Can you work these out from the model? Positions are in its coordinate system, mm. A direction names the side the tool comes from. Give positions to 0.01 mm unless a question says otherwise; leave off trailing zeros. Order: outer loops, then holes, each group sorted by start corner. A loop starts at its lowest first (then second) coordinate and runs counter-clockwise, first axis right, second up. Notation, with made-up numbers: (-5.5, -15) - (46.5, -15) arc R10 ccw to (46.5, -11) - close; hole circle Ø2 at (43, -15). An arc over 180 degrees is marked (long way). Return JSON: item names as keys, results as strings.
```python
from build123d import *

# Parameters (mm, degrees)
SKETCH_W      = 50
SKETCH_H      = 53
PAD_DEPTH     = 3
SKETCH001_W   = 50
SKETCH001_H   = 3
PAD001_DEPTH  = 48
SKETCH002_R   = 11.05
SKETCH002_R_2 = 1.75
POCKET_DEPTH  = 53.001
FILLET_R      = 2
CHAMFER_SIZE  = 5


with BuildPart() as part:
    # Sketch → Pad (new body)
    with BuildSketch(Plane.XY):
        Rectangle(SKETCH_W, SKETCH_H)
        with BuildLine():
            ThreePointArc((-17.1, -15.5), (-15, -17.6), (-12.9, -15.5))
            Line((-12.9, -15.5), (-12.9, 14.5))
            ThreePointArc((-12.9, 14.5), (-15, 16.6), (-17.1, 14.5))
            Line((-17.1, -15.5), (-17.1, 14.5))
        make_face(mode=Mode.SUBTRACT)
        with BuildLine():
            ThreePointArc((12.9, -15.5), (15, -17.6), (17.1, -15.5))
            Line((17.1, -15.5), (17.1, 14.5))
            ThreePointArc((17.1, 14.5), (15, 16.6), (12.9, 14.5))
            Line((12.9, -15.5), (12.9, 14.5))
        make_face(mode=Mode.SUBTRACT)
    extrude(amount=PAD_DEPTH)

    # Sketch001 → Pad001 (new body)
    with BuildSketch(Plane.XY.offset(3)):
        with Locations((0, 25)):
            Rectangle(SKETCH001_W, SKETCH001_H)
    extrude(amount=PAD001_DEPTH)

    # Sketch002 → Pocket (cut, through all)
    with BuildSketch(Plane(origin=(0, 26.5, 0), x_dir=(-1, 0, 0), z_dir=(0, 1, 0))):
        with Locations((0, 30)):
            Circle(SKETCH002_R)
        with Locations((-15.5, 45.5)):
            Circle(SKETCH002_R_2)
        with Locations((15.5, 45.5)):
            Circle(SKETCH002_R_2)
        with Locations((-15.5, 14.5)):
            Circle(SKETCH002_R_2)
        with Locations((15.5, 14.5)):
            Circle(SKETCH002_R_2)
    extrude(amount=-POCKET_DEPTH, mode=Mode.SUBTRACT)

    # Fillet
    fillet_edges = [part.edges().sort_by_distance(p)[0] for p in [
        (0, 26.5, 0),
        (0, 23.5, 3),
    ]]
    fillet(fillet_edges, radius=FILLET_R)

    # Chamfer
    chamfer_edges = [part.edges().sort_by_distance(p)[0] for p in [
        (25, 25, 51),
        (-25, 25, 51),
        (-25, -26.5, 1.5),
        (25, -26.5, 1.5),
    ]]
    chamfer(chamfer_edges, length=CHAMFER_SIZE)


solid = part.part
```
1. Suppose I cut it at D-D (x = 12). List the corners of the cut face in (y, z) for me.
Checks:
{"outline": "(-26.5, 0) - (24.5, 0) arc R2 ccw to (26.5, 2) - (26.5, 51) - (23.5, 51) - (23.5, 5) arc R2 cw to (21.5, 3) - (-26.5, 3) - close"}
2. Thinking about a two-plate mould opening in Z: for faces 1 (the face through (23, 25, 48)), 2 (the face through (-15, 16.6, 1.5)), 3 (the face through (-15.12, 25.02, 43.79)), which applies, +Z half, -Z half, draft (parallel to the pull), parting line (faces both ways), or undercut?
Checks:
{"face 1": "+Z half", "face 2": "draft", "face 3": "undercut"}
3. Suppose I cut it at B-B (y = 2.5). List the corners of the cut face in (x, z) for me.
Checks:
{"outline": "(-25, 0) - (-17.1, 0) - (-17.1, 3) - (-25, 3) - close; (-12.9, 0) - (12.9, 0) - (12.9, 3) - (-12.9, 3) - close; (17.1, 0) - (25, 0) - (25, 3) - (17.1, 3) - close"}
4. Suppose I cut it at C-C (z = 14.5). List the corners of the cut face in (x, y) for me, plus the area to 3 significant figures.
Checks:
{"outline": "(-25, 23.5) - (-17.25, 23.5) - (-17.25, 26.5) - (-25, 26.5) - close; (-13.75, 23.5) - (13.75, 23.5) - (13.75, 26.5) - (-13.75, 26.5) - close; (17.25, 23.5) - (25, 23.5) - (25, 26.5) - (17.25, 26.5) - close", "area": "129 mm^2"}
5. For pin 1 Ø1.5 at (x, y) = (-8.5, 13.5) entering from +Z; pin 2 Ø5.5 at (x, z) = (-15.5, 14.5) entering from -Y; pin 3 Ø3 at (x, z) = (15.5, 14.5) entering from -Y, each with a flat end and sliding along its axis, tell me the tip position at first contact or that it passes through.
Checks:
{"pin 1": "z = 3", "pin 2": "y = 23.5", "pin 3": "through"}
6. On a 3-axis mill with a long thin cutter (end or side, diameter ignored), from which of +Z, -Z, +X, -X, +Y, -Y can I reach the whole of each face in a straight line? I mean faces 4 (the face through (0, -2, 3)), 5 (the face through (-17.1, -1, 1)), 6 (the face through (-25, 13, 2)). Say none if no direction works.
Checks:
{"face 4": "+Z, +X, -X, -Y", "face 5": "+Z, -Z", "face 6": "+Z, -Z, -X, +Y, -Y"}
7. Suppose I cut it at A-A (x = 0). List the corners of the cut face in (y, z) for me, plus the area to 3 significant figures.
Checks:
{"outline": "(-26.5, 0) - (24.5, 0) arc R2 ccw to (26.5, 2) - (26.5, 18.95) - (23.5, 18.95) - (23.5, 5) arc R2 cw to (21.5, 3) - (-26.5, 3) - close; (23.5, 41.05) - (26.5, 41.05) - (26.5, 51) - (23.5, 51) - close", "area": "237 mm^2"}
8. If I drill on L1, parallel to Z at x = -15.5, y = 24.45; L2, parallel to Z at x = -15.5, y = 25.7; L3, parallel to Y at x = 5, z = 7, over which ranges is the centre line in solid material (lowest first)? Write a range as [from, to].
Checks:
{"L1": "[0, 12.75], [16.25, 43.75], [47.25, 51]", "L2": "[0.4, 12.75], [16.25, 43.75], [47.25, 51]", "L3": "[23.5, 26.5]"}
